from build123d import *

# Parameters (mm, degrees)
CROQUIS1_R              = 57.15
CROQUIS1_R_2            = 51.15
SALIENTE_EXTRUIR1_DEPTH = 580
CORTAR_EXTRUIR1_START   = -101.6
CORTAR_EXTRUIR1_DEPTH   = 101.6


with BuildPart() as part:
    # Croquis1 → Saliente-Extruir1 (new body)
    with BuildSketch(Plane(origin=(0, 0, 0), x_dir=(0, 0, -1), z_dir=(1, 0, 0))):
        Circle(CROQUIS1_R)
        Circle(CROQUIS1_R_2, mode=Mode.SUBTRACT)
    extrude(amount=SALIENTE_EXTRUIR1_DEPTH)

    # Croquis2 → Cortar-Extruir1 (cut)
    with BuildSketch(Plane(origin=(580, 0, 0), x_dir=(0, 0, -1), z_dir=(1, 0, 0)).offset(CORTAR_EXTRUIR1_START)):
        with BuildLine():
            Line((-48.140237847, -30.8), (48.140237847, -30.8))
            ThreePointArc((48.140237847, -30.8), (0, -57.15), (-48.140237847, -30.8))
        make_face()
    extrude(amount=CORTAR_EXTRUIR1_DEPTH, mode=Mode.SUBTRACT)


solid = part.part
The listing builds one solid part. Answer for the finished solid, in the listing's coordinates (mm). A direction names the side the tool comes from. Coordinates: 2 decimals unless noted, no trailing zeros. Loops run counter-clockwise (first coordinate to the right, second up) from the corner with the lowest first, then second, coordinate; pieces in that order, holes last.
1) Find section A-A on z = 0. Write down the section's boundary in (x, y), then the cut area to 3 significant figures.
2) Flat-ended cylindrical pins translate along their axes: pin 1 Ø1.5 at (x, z) = (392.5, -20.5) entering from -Y; pin 2 Ø1 at (x, y) = (412, -15.5) entering from -Z; pin 3 Ø8 at (x, z) = (515, 45.5) entering from -Y; pin 4 Ø10 at (y, z) = (45, 43.5) entering from -X. Find the tip coordinate at first contact, or state that the pin passes through.
3) Find section B-B on y = 0. Write down the section's boundary in (x, z).
4) Find section C-C on x = 123. Write down the section's boundary in (y, z), then the cut area to 3 significant figures.
5) A tool of negligible diameter and unlimited length cuts with its end or side. For faces 1 (the face through (580, 52, 0)), 2 (the face through (478.4, -53, 0)), from which of +Z, -Z, +X, -X, +Y, -Y can it reach the whole face along a straight path? Write none if from no direction.
6) Determine the mould class of faces 3 (the face through (285.94, 56.664, 7.44)), 4 (the face through (285.94, 43.13, -27.5)), 5 (the face through (0, -29, 43)) for opening direction Z: pulls with the +Z half, pulls with the -Z half, needs draft (parallel to the pull), parting line crosses it, or undercut.
7) Find the intervals of material crossed by L1, parallel to Y at x = 151.5, z = 0; L2, parallel to Z at x = 220, y = 41.5; L3, parallel to Z at x = 373.5, y = -45, in increasing order.
Values:
1. outline: (0, -57.15) - (478.4, -57.15) - (478.4, -51.15) - (0, -51.15) - close; (0, 51.15) - (580, 51.15) - (580, 57.15) - (0, 57.15) - close
1. area: 6,350 mm2
2. pin 1: stops at y = -53.63
2. pin 2: stops at z = -55.15
2. pin 3: stops at y = -30.8
2. pin 4: passes through
3. outline: (0, -57.15) - (580, -57.15) - (580, -51.15) - (0, -51.15) - close; (0, 51.15) - (580, 51.15) - (580, 57.15) - (0, 57.15) - close
4. outline: circle Ø114.3 at (0, 0); hole circle Ø102.3 at (0, 0)
4. area: 2,040 mm2
5. face 1: +Z, -Z, +X, +Y, -Y
5. face 2: +Z, -Z, +X, -Y
6. face 3: parting line crosses it
6. face 4: undercut
6. face 5: needs draft
7. L1: y = -57.15 to -51.15, 51.15 to 57.15
7. L2: z = -39.29 to -29.9, 29.9 to 39.29
7. L3: z = -35.23 to -24.32, 24.32 to 35.23
